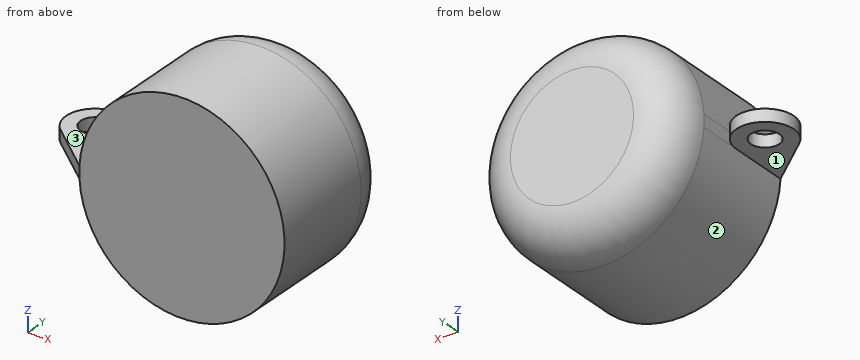
```python
from build123d import *

# Parameters (mm, degrees)
SKETCH5_W                            = 3
SKETCH5_H                            = 26
BOSS_EXTRUDE1_DEPTH                  = 15
BOSS_EXTRUDE1_DIRECTION_2_REACH      = 68.491
BOSS_EXTRUDE1_DIRECTION_2_END_RADIUS = 25
CUT_EXTRUDE1_DEPTH                   = 60.338014797
CUT_EXTRUDE1_DEPTH_BACK              = 60.338014797
SKETCH4_R                            = 3.5


with BuildPart() as part:
    # Sketch1 → Revolve1 (revolve)
    with BuildSketch(Plane.XY, mode=Mode.PRIVATE) as revolve1_sk:
        with BuildLine():
            Line((0, 0), (25, 0))
            Line((25, 0), (25, 26))
            ThreePointArc((25, 26), (22.071067812, 33.071067812), (15, 36))
            Line((15, 36), (0, 36))
            Line((0, 36), (0, 35))
            Line((0, 35), (1, 35))
            Line((1, 35), (15, 35))
            ThreePointArc((15, 35), (21.363961031, 32.363961031), (24, 26))
            Line((24, 26), (24, 1))
            Line((24, 1), (1, 1))
            Line((1, 1), (0, 1))
            Line((0, 1), (0, 0))
        make_face()
    revolve(revolve1_sk.sketch.rotate(Axis((0, 36, 0), (0, -1, 0)), 180), axis=Axis((0, 36, 0), (0, -1, 0)))

    # Sketch5 → Boss-Extrude1 (add)
    with BuildSketch(Plane.ZY.offset(25)):
        with Locations((0, 13)):
            Rectangle(SKETCH5_W, SKETCH5_H)
    extrude(amount=BOSS_EXTRUDE1_DEPTH)

    # Boss-Extrude1 direction 2: up to this cylinder (the profile starts outside it)
    boss_extrude1_direction_2_end = Plane(origin=(0, 13, 0), z_dir=(0, 1, 0)) * Cylinder(BOSS_EXTRUDE1_DIRECTION_2_END_RADIUS, 187.982, mode=Mode.PRIVATE)
    # Sketch5 → Boss-Extrude1 direction 2 (add, up to the surface)
    with BuildSketch(Plane.ZY.offset(25), mode=Mode.PRIVATE) as boss_extrude1_direction_2_sk1:
        with Locations((0, 13)):
            Rectangle(SKETCH5_W, SKETCH5_H)
    boss_extrude1_direction_2_tool1 = extrude(boss_extrude1_direction_2_sk1.sketch, amount=-BOSS_EXTRUDE1_DIRECTION_2_REACH, mode=Mode.PRIVATE) - boss_extrude1_direction_2_end
    add(boss_extrude1_direction_2_tool1.solids().sort_by_distance((-25, 13, 0))[0])
    add(boss_extrude1_direction_2_tool1.solids().sort_by_distance((-25, 13, 0))[1])

    # Sketch4 → Cut-Extrude1 (cut, two sides: drawn at the far end of the back side and taken through both)
    with BuildSketch(Plane.XY.offset(-CUT_EXTRUDE1_DEPTH_BACK)):
        with Locations(Location((-31.954959427, 15, 0), (0, 0, 90))):
            Circle(SKETCH4_R)
        with BuildLine():
            Line((-24.954959427, 0), (-36.451309792, 9.635036496))
            ThreePointArc((-36.451309792, 9.635036496), (-34.915157684, 21.34328198), (-24.954959427, 15))
            Line((-24.954959427, 15), (-24.954959427, 26))
            Line((-24.954959427, 26), (-40, 26))
            Line((-40, 26), (-40, 0))
            Line((-40, 0), (-24.954959427, 0))
        make_face()
    extrude(amount=CUT_EXTRUDE1_DEPTH + CUT_EXTRUDE1_DEPTH_BACK, mode=Mode.SUBTRACT)


solid = part.part
```
Design review of the part built by this model. Coordinates are the model's own, in mm. Face numbers are marked on the shaded views. A direction names the side the tool comes from. Give positions to 0.01 mm unless a question says otherwise; leave off trailing zeros. Order: outer loops, then holes, each group sorted by start corner. A loop starts at its lowest first (then second) coordinate and runs counter-clockwise, first axis right, second up. Notation, with made-up numbers: (27, 2.25) -> (49, 2.25) arc R25 ccw to (49, 25.25) -> close; hole circle Ø7 at (77.5, 13). An arc over 180 degrees is marked (long way). Write item = value, one per line. Start each with the question number.
(1) We need section C-C on z = 0. Write out the cut boundary in (x, y).
(2) We need section B-B on y = 21. Write out the cut boundary in (x, z), plus the area to 3 significant figures.
(3) To check wall thickness, follow line 1 along Z through (x, y) = (-0.5, 16) (3 decimals); line 2 along Y through (x, z) = (6, -5); line 3 along X through (y, z) = (7, 17). State the ranges of each line that lie inside material, in increasing order.
(4) We need section D-D on y = 3.5. Write out the cut boundary in (x, z), plus the area to 3 significant figures.
(5) For the marked faces 1, 2 and 3, list the 3-axis set-ups (+Z, -Z, +X, -X, +Y, -Y) from which the entire face can be reached by the end or side of a thin tool; tool diameter is ignored.
(6) For pin 1 (1 mm diameter, centred on x = -16.5, y = 12, fed in from +Z); pin 2 (5 mm diameter, centred on x = -7, y = 23.5, fed in from -Z); pin 3 (0.9 mm diameter, centred on y = 23, z = 0.5, fed in from -X), all flat-tipped, find the tip position at first contact; note any pin that passes through.
(7) We need section A-A on x = 0. Write out the cut boundary in (y, z).
Numbers:
q1.outline = (-36.45, 9.64) -> (-24.95, 0) -> (25, 0) -> (25, 26) arc R10 ccw to (15, 36) -> (-15, 36) arc R10 ccw to (-25, 26) -> (-24.95, 26) -> (-24.95, 15) arc R7 ccw (long way) to start; hole circle Ø7 at (-31.95, 15); hole (-24, 1) -> (24, 1) -> (24, 26) arc R9 ccw to (15, 35) -> (-15, 35) arc R9 ccw to (-24, 26) -> close
q2.outline = (-35.56, -1.5) -> (-28.35, -1.5) -> (-28.35, 1.5) -> (-35.56, 1.5) -> close; (-24.95, -1.5) arc R25 ccw (long way) to (-24.95, 1.5) -> close; hole circle Ø48 at (0, 0)
q2.area = 175 mm^2
q3.line_1 = -24.995 to -23.995, 23.995 to 24.995
q3.line_2 = 0 to 1, 35 to 36
q3.line_3 = -18.33 to -16.94, 16.94 to 18.33
q4.outline = (-29.13, -1.5) -> (-24.95, -1.5) arc R25 ccw (long way) to (-24.95, 1.5) -> (-29.13, 1.5) -> close; hole circle Ø48 at (0, 0)
q4.area = 166 mm^2
q5.face_1 = -Z, -X, +Y, -Y
q5.face_2 = +Y, -Y
q5.face_3 = +Z, -X, +Y, -Y
q6.pin_1 = 19.21
q6.pin_2 = -24.59
q6.pin_3 = -24.95
q7.outline = (0, -25) -> (26, -25) arc R10 ccw to (36, -15) -> (36, 15) arc R10 ccw to (26, 25) -> (0, 25) -> close; hole (1, -24) -> (26, -24) arc R9 ccw to (35, -15) -> (35, 15) arc R9 ccw to (26, 24) -> (1, 24) -> close
